Geometry check sheet. Reference: drawing and pictorial views, mm from the part's lowest x, y, z. A direction names the side the tool comes from. Give positions to 0.01 mm unless a question says otherwise; leave off trailing zeros. Order: outer loops, then holes, each group sorted by start corner. A loop starts at its lowest first (then second) coordinate and runs counter-clockwise, first axis right, second up. Notation, with made-up numbers: (48.5, 40) - (80.5, 40) arc R11 cw to (80.5, 55) - close; hole circle Ø9 at (35, -7.75). An arc over 180 degrees is marked (long way). Answer in a Markdown table with one row per item.
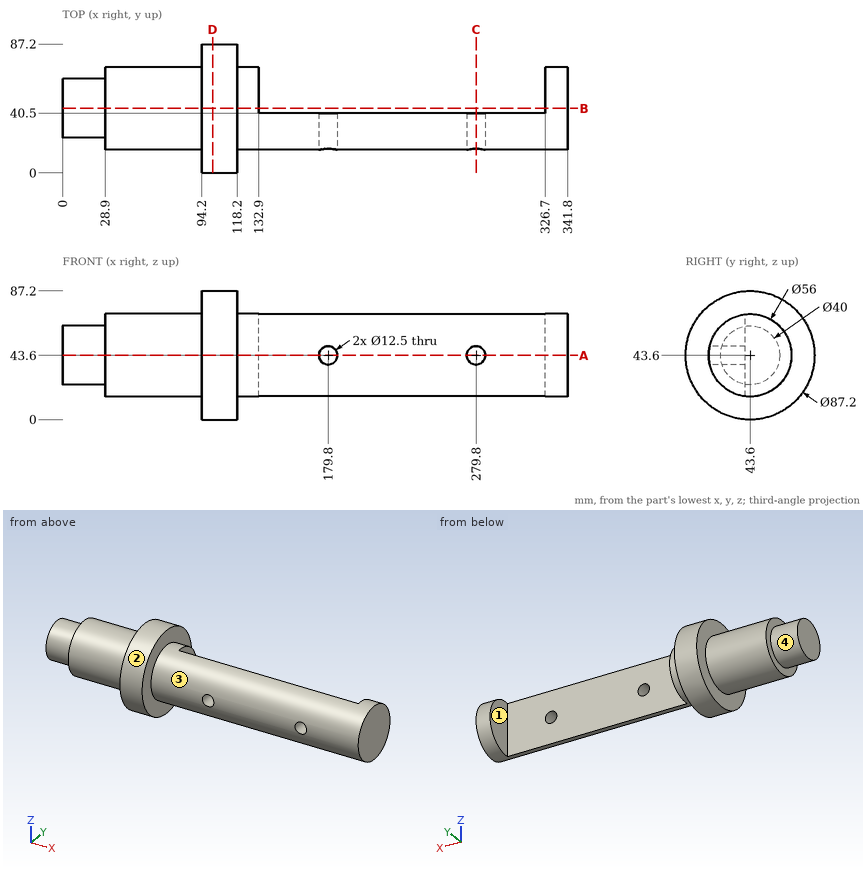
(1) Cross-section at B-B, the plane y = 43.6. Record the cut outline in (x, z).
Geometry says:
| item | result |
|---|---|
| outline | (0, 23.6) - (28.9, 23.6) - (28.9, 15.6) - (94.2, 15.6) - (94.2, 0) - (118.2, 0) - (118.2, 15.6) - (132.9, 15.6) - (132.9, 71.6) - (118.2, 71.6) - (118.2, 87.2) - (94.2, 87.2) - (94.2, 71.6) - (28.9, 71.6) - (28.9, 63.6) - (0, 63.6) - close; (326.7, 15.6) - (341.8, 15.6) - (341.8, 71.6) - (326.7, 71.6) - close |
(2) Cross-section at D-D, the plane x = 101.5. Record the cut outline in (y, z).
Geometry says:
| item | result |
|---|---|
| outline | circle Ø87.2 at (43.6, 43.6) |
(3) Gauge pin test, flat ends, axial feed: P1, Ø1.5, axis at x = 193, z = 23, coming from the +Y side; P2, Ø8, axis at x = 103, y = 52, coming from the +Z side; P3, Ø10, axis at x = 104.5, z = 38, coming from the -Y side. Record the tip position at first contact, or that the pin passes through.
Geometry says:
| item | result |
|---|---|
| P1 | y = 40.5 |
| P2 | z = 86.98 |
| P3 | y = 0 |
(4) Cross-section at C-C, the plane x = 279.8. Record the cut outline in (y, z), then the cut area to 3 significant figures.
Geometry says:
| item | result |
|---|---|
| outline | (16.31, 37.35) arc R28 ccw to (40.5, 15.77) - (40.5, 37.35) - close; (16.31, 49.85) - (40.5, 49.85) - (40.5, 71.43) arc R28 ccw to start |
| area | 750 mm² |
(5) Access from +Z, -Z, +X, -X, +Y, -Y to the whole of each face (thin tool, end or side, straight path). Record for the marked faces 1, 2, 3 and 4.
Geometry says:
| item | result |
|---|---|
| face 1 | +Z, -Z, +Y |
| face 2 | +X, -X |
| face 3 | +X |
| face 4 | -X |
(6) Cross-section at A-A, the plane z = 43.6. Record the cut outline in (x, y).
Geometry says:
| item | result |
|---|---|
| outline | (0, 23.6) - (28.9, 23.6) - (28.9, 15.6) - (94.2, 15.6) - (94.2, 0) - (118.2, 0) - (118.2, 15.6) - (173.55, 15.6) - (173.55, 40.5) - (132.9, 40.5) - (132.9, 71.6) - (118.2, 71.6) - (118.2, 87.2) - (94.2, 87.2) - (94.2, 71.6) - (28.9, 71.6) - (28.9, 63.6) - (0, 63.6) - close; (186.05, 15.6) - (273.55, 15.6) - (273.55, 40.5) - (186.05, 40.5) - close; (286.05, 15.6) - (341.8, 15.6) - (341.8, 71.6) - (326.7, 71.6) - (326.7, 40.5) - (286.05, 40.5) - close |
(7) Thickness scan on L1, parallel to X at y = 35, z = 43.6; L2, parallel to X at y = 61, z = 22; L3, parallel to X at y = 15, z = 43.5. Record the ranges inside material, lowest first.
Geometry says:
| item | result |
|---|---|
| L1 | 0 to 173.55, 186.05 to 273.55, 286.05 to 341.8 |
| L2 | 28.9 to 132.9, 326.7 to 341.8 |
| L3 | 94.2 to 118.2 |
